```python
from build123d import *

# Parameters (mm, degrees)
ESBO_O1_W                = 80
ESBO_O1_H                = 20
RESSALTO_EXTRUS_O1_DEPTH = 3
ESBO_O2_R                = 10
CORTE_EXTRUS_O1_DEPTH    = 10
FILETE1_R                = 0.8
FILETE2_R                = 0.8


with BuildPart() as part:
    # Esboço1 → Ressalto-extrusão1 (new body)
    with BuildSketch(Plane.XY):
        with Locations((-5.941010257, 18.311759729)):
            Rectangle(ESBO_O1_W, ESBO_O1_H)
    extrude(amount=RESSALTO_EXTRUS_O1_DEPTH)

    # Esboço2 → Corte-extrusão1 (cut)
    with BuildSketch(Plane.XY.offset(3)):
        with Locations((34.058989743, 18.311759729)):
            Circle(ESBO_O2_R)
    extrude(amount=-CORTE_EXTRUS_O1_DEPTH, mode=Mode.SUBTRACT)

    # Filete1
    filete1_edges = [part.edges().sort_by_distance(p)[0] for p in [
        (34.058989743, 28.311759729, 1.5),
    ]]
    fillet(filete1_edges, radius=FILETE1_R)

    # Filete2
    # the kernel refuses this fillet: 0.8 mm, written as the material it takes off along each edge
    with BuildSketch(Plane(origin=(34.058989743, 8.311759729, -14.142135624), x_dir=(-0.9622504486493761, 0.2721655269759089, 0), z_dir=(0, 0, 1))) as filete2_piece_1:
        with BuildLine():
            CenterArc((5.661042961, 0.769800359), FILETE2_R, 105.793169048, 148.413661903)
            Line((5.44331054, 1.539600718), (0, 0))
            ThreePointArc((0, 0), (2.72165527, 0.377495514), (5.44331054, 0))
        make_face()
    extrude(amount=31.284271247, mode=Mode.SUBTRACT)


solid = part.part
```
Geometry check sheet. Reference: the model listing, model coordinates, mm. Coordinates: 2 decimals unless noted, no trailing zeros. Write each loop counter-clockwise with the first axis right and the second up, starting at its lowest first coordinate (ties: lowest second). Pieces come first, ordered by that corner, then holes. Notation, with made-up numbers: (65.5, 6.5) -> (98.5, 6.5) arc R16 cw to (98.5, 19.5) -> close; hole circle Ø11 at (78, -17.75). An arc over 180 degrees is marked (long way). Use CSV: the item, a comma, the result in double quotes. Start each with the question number.
Item 1: Depth check by flat-ended pin: pin 1 Ø1 at (y, z) = (23, 2.5) entering from +X. Enter the tip coordinate at first touch or a pass-through.
Item 2: Cross-section at B-B, the plane y = 14.5. Record the cut outline in (x, z).
Item 3: Cross-section at A-A, the plane z = 1.75. Record the cut outline in (x, y), plus the area to 3 significant figures.
Item 4: Mould release check, pull along Y, two halves, no side actions. Record for faces 1 (the cylindrical face through (24.06, 18.45, 1.52)), 2 (the cylindrical face through (29.17, 27.74, 1.52)), 3 (the flat face through (-9, 28.312, 1)), 4 (the flat face through (-9, 18, 0)): released by +Y, released by -Y, zero draft, split by the parting line, or undercut.
Item 5: Thickness scan on line 1 (X direction, y = 18.5, z = 2.25); line 2 (Y direction, x = 26.5, z = 1); line 3 (X direction, y = 14.75, z = 1.1). Record the ranges inside material, lowest first.
Item 6: Cross-section at C-C, the plane y = 24.5. Record the cut outline in (x, z).
Answers:
1,pin 1,"x = 25.51"
2,outline,"(-45.94, 0) -> (24.81, 0) -> (24.81, 3) -> (-45.94, 3) -> close"
3,outline,"(-45.94, 8.31) -> (28.4, 8.31) arc R0.8 ccw to (28.82, 9.79) arc R10 cw to (28.82, 26.83) arc R0.8 ccw to (28.4, 28.31) -> (-45.94, 28.31) -> close"
3,area,"1,440 mm^2"
4,face 1,"undercut"
4,face 2,"undercut"
4,face 3,"released by +Y"
4,face 4,"zero draft"
5,line 1,"-45.94 to 24.06"
5,line 2,"8.31 to 11.76, 24.86 to 28.31"
5,line 3,"-45.94 to 24.71"
6,outline,"(-45.94, 0) -> (26.2, 0) -> (26.2, 3) -> (-45.94, 3) -> close"
